The listing builds one solid part. Answer for the finished solid, in the listing's coordinates (mm). Round coordinates to 2 decimals unless told otherwise and drop trailing zeros. Write each loop counter-clockwise with the first axis right and the second up, starting at its lowest first coordinate (ties: lowest second). Pieces come first, ordered by that corner, then holes.
(1) A cutting plane is placed at A-A, the plane z = 0. Give the vertices of the cut face in (x, y), and give its area (3 significant figures).
(2) Find the intervals of material crossed by probe 1 along Y at (x, z) = (-1.25, -0.65); probe 2 along Y at (x, z) = (-2, -1.3); probe 3 along X at (y, z) = (-0.25, 0.65), in increasing order.
(3) A cutting plane is placed at B-B, the plane x = -1.25. Give the vertices of the cut face in (y, z).
(4) This flat-tipped pin is pushed along its axis until it touches: pin 1 Ø1.5 at (y, z) = (0.5, 0) entering from +X. Where does it stop, or does it pass through?
(5) A cutting plane is placed at C-C, the plane y = -0.55. Give the vertices of the cut face in (x, z), and give its area (3 significant figures).
(6) A cutting plane is placed at D-D, the plane z = -0.35. Give the vertices of the cut face in (x, y), and give its area (3 significant figures).
from build123d import *

# Parameters (mm, degrees)
CIRPATTERN1_COUNT = 3


with BuildPart() as part:
    # Sketch1 → Base-Revolve (revolve)
    with BuildSketch(Plane.XY):
        with BuildLine():
            Line((-4, 0), (-4, 0.15))
            ThreePointArc((-4, 0.15), (-3.881206061, 0.848681403), (-3.601828558, 1.5))
            Line((-3.601828558, 1.5), (3.598076211, 1.5))
            ThreePointArc((3.598076211, 1.5), (3.897777479, 0.776457135), (4, 0))
            Line((4, 0), (-4, 0))
        make_face()
    revolve(axis=Axis((-57, 0, 0), (1, 0, 0)))

    # Cut-Sweep1: sweep along a path in Sketch3
    with BuildLine(Plane(origin=(0, 0, 0), x_dir=(1, 0, 0), z_dir=(0, 1, 0))) as cut_sweep1_path:
        Line((0, -1.5), (0.375, -1.35))
        Line((0.375, -1.35), (4, -1.5))
    # Sketch2 → Cut-Sweep1 (sweep, cut)
    with BuildSketch(Plane(origin=(0, 0, 0), x_dir=(0, 0, -1), z_dir=(1, 0, 0))):
        Polygon((-1.5, 0), (-3.378358908, 1.315241067), (-3.378358908, -1.315241067), align=None)
    cut_sweep1 = sweep(path=cut_sweep1_path.line, transition=Transition.RIGHT, mode=Mode.SUBTRACT)

    # CirPattern1: Cut-Sweep1 ×3 about axis
    cirpattern1_axis = Axis((0, 0, 0), (1, 0, 0))
    for i in range(1, CIRPATTERN1_COUNT):
        add(cut_sweep1.rotate(cirpattern1_axis, i * 360 / CIRPATTERN1_COUNT), mode=Mode.SUBTRACT)


solid = part.part
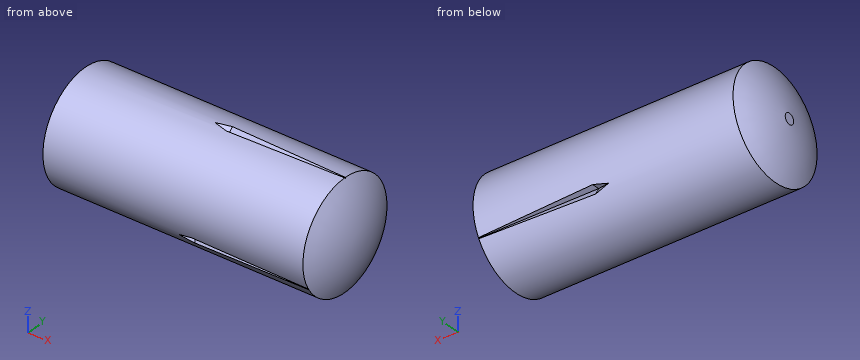
Solutions:
1. outline: (-4, -0.15) arc R3 ccw to (-3.6, -1.5) - (3.6, -1.5) arc R3 ccw to (3.6, 1.5) - (-3.6, 1.5) arc R3 ccw to (-4, 0.15) - close
1. area: 23.2 mm2
2. probe 1: y = -1.35 to 1.35
2. probe 2: y = -0.75 to 0.75
2. probe 3: x = -3.92 to 3.92
3. outline: circle Ø3 at (0, 0)
4. pin 1: stops at x = 4
5. outline: (-3.6, -1.4) - (3.6, -1.4) arc R2.95 ccw to (3.6, 1.4) - (-3.6, 1.4) arc R2.95 ccw to start
5. area: 21.4 mm2
6. outline: (-3.6, -1.46) - (3.6, -1.46) arc R2.98 ccw to (3.6, 1.46) - (-3.6, 1.46) arc R2.98 ccw to start
6. area: 22.5 mm2
